Autodesk Inventor part; units mm, degrees
ref_plane "YZ Plane" through (0, 0, 0) normal (1, 0, 0) x (0, 1, 0)
ref_plane "XZ Plane" through (0, 0, 0) normal (0, 1, 0) x (-1, 0, 0)
ref_plane "XY Plane" through (0, 0, 0) normal (0, 0, 1) x (1, 0, 0)
sketch "Schizzo1" plane through (0, 0, 0) normal (0, 0, 1) x (1, 0, 0)
  line L0 (9, 6) -> (9, -6)
  line L1 (6, -9) -> (-6, -9)
  line L2 (-9, -6) -> (-9, 6)
  line L3 (-6, 9) -> (6, 9)
  arc A0 (-6, 9) -> (-9, 6) centre (-6, 6) ccw
  arc A1 (-9, -6) -> (-6, -9) centre (-6, -6) ccw
  arc A2 (6, -9) -> (9, -6) centre (6, -6) ccw
  arc A3 (9, 6) -> (6, 9) centre (6, 6) ccw
  point P0 (0, 0)
  point P1 (0, 0)
  point P2 (9, 9)
  point P3 (9, -9)
  point P4 (-9, -9)
  point P5 (-9, 9)
  dimension "d0" = 18
  dimension "d72" = 3
extrude "Estrusione1" add sketch "Schizzo1" against normal blind 40
sketch "Schizzo2" plane through (0, 0, 0) normal (0, 0, 1) x (1, 0, 0)
  line L0 (18.5, -15) -> (-18.5, -15)
  line L1 (-18.5, -15) -> (-18.5, 15)
  line L2 (-18.5, 15) -> (18.5, 15)
  line L3 (18.5, 15) -> (18.5, -15)
  line L4 (18.5, -15) -> (-18.5, 15) construction
  line L5 (-18.5, -15) -> (18.5, 15) construction
  point P0 (0, 0)
  dimension "d3" = 30
  dimension "d4" = 37
extrude "Estrusione2" add sketch "Schizzo2" along normal blind 50
sketch "Schizzo3" plane through (-18.5, 15, 0) normal (0, 1, 0) x (1, 0, 0)
  line L0 (18.5, 0) -> (18.5, -22.5)
  line L1 (18.5, 0) -> (41, 0) construction
  circle A0 centre (18.5, -22.5) radius 12.5
  dimension "d7" = 22.5
  dimension "d8" = 90
  dimension "d9" = 25
extrude "Estrusione3" cut sketch "Schizzo3" against normal blind 30
sketch "Schizzo4" plane through (-18.5, 15, 0) normal (0, 1, 0) x (1, 0, 0)
  circle A0 centre (18.5, -22.5) radius 12.5
  line L0 (18.5, -22.5) -> (18.5, -34.5)
  line L1 (18.5, -34.5) -> (15, -34.5)
  line L2 (18.5, -34.5) -> (22, -34.5)
  line L3 (0, -50) -> (37, -50)
  line L4 (18.5, -50) -> (20.5, -50)
  line L5 (18.5, -50) -> (20.5, -50) construction
  line L6 (20.5, -50) -> (20.5, -34.5)
  line L7 (18.5, -50) -> (16.5, -50)
  line L8 (16.5, -50) -> (20.5, -50)
  line L9 (20.5, -50) -> (20.5, -34.5)
  line L10 (20.5, -34.5) -> (16.5, -34.5)
  line L11 (16.5, -34.5) -> (16.5, -50)
  point P0 (18.5, 0)
  point P1 (16.5, -34.839)
  point P2 (20.5, -34.839)
  dimension "d12" = 12
  dimension "d13" = 2
  dimension "d14" = 0
  dimension "d15" = 2
extrude "Estrusione4" cut sketch "Schizzo4" against normal blind 30 contours A0 L6 L3 L11
sketch "Schizzo5" plane through (-18.5, 15, 0) normal (0, 1, 0) x (1, 0, 0)
  arc A0 (20.5, -34.839) -> (16.5, -34.839) centre (18.5, -22.5) ccw
  circle A1 centre (18.5, -22.5) radius 18.5
  line L0 (20.5, -50) -> (20.5, -34.839)
  line L1 (20.5, -50) -> (26.5, -50)
  line L2 (37, -50) -> (20.5, -50)
  line L3 (26.5, -50) -> (26.5, -39.1808)
  line L4 (37, 0) -> (37, -50)
  line L5 (26.5, -50) -> (37, -50)
  line L6 (37, -50) -> (37, -22.5)
  point P0 (18.5, 0)
  dimension "d18" = 37
  dimension "d19" = 6
extrude "Estrusione5" cut sketch "Schizzo5" against normal blind 30 contours A1 L4 L2 L3
sketch "Schizzo6" plane through (-18.5, 15, 0) normal (0, 1, 0) x (1, 0, 0)
  line L0 (16.5, -50) -> (0, -50)
  line L1 (16.5, -50) -> (10.5, -50)
  arc A0 (20.5, -34.839) -> (16.5, -34.839) centre (18.5, -22.5) ccw
  circle A1 centre (18.5, -22.5) radius 18.5
  line L2 (0, 0) -> (0, -50)
  line L3 (10.5, -50) -> (0, -50)
  line L4 (0, -50) -> (0, -22.5)
  line L5 (10.5, -50) -> (10.5, -39.1808)
  line L6 (10.5, -50) -> (21.3192, -50) construction
  point P0 (18.5, 0)
  dimension "d22" = 6
  dimension "d23" = 37
  dimension "d24" = 90
extrude "Estrusione6" cut sketch "Schizzo6" against normal blind 30 contours L0 L2 A1 L5
sketch "Schizzo7" plane through (-18.5, 15, 0) normal (0, 1, 0) x (1, 0, 0)
  arc A0 (20.5, -34.839) -> (16.5, -34.839) centre (18.5, -22.5) ccw
  line L0 (0, 0) -> (0, -22.5)
  circle A1 centre (18.5, -22.5) radius 18.5
  line L1 (18.5, 0) -> (4.5, 0)
  line L2 (37, 0) -> (0, 0)
  line L3 (18.5, 0) -> (32.5, 0) construction
  line L4 (4.5, 0) -> (4.5, -10.4066)
  dimension "d73" = 37
  dimension "d74" = 14
  dimension "d75" = 180
  dimension "d76" = 90
extrude "Estrusione7" cut sketch "Schizzo7" against normal blind 30 contours L2 L4 A1 L0
sketch "Schizzo8" plane through (0, 15, 22.5) normal (0, 1, 0) x (1, 0, 0)
  line L0 (-6, 22.5) -> (6, 22.5)
  arc A0 (2, -12.339) -> (-2, -12.339) centre (0, 0) ccw
  circle A1 centre (0, 0) radius 18.5
  line L1 (0, 22.5) -> (14, 22.5)
  line L2 (0, 22.5) -> (14, 22.5) construction
  line L3 (14, 22.5) -> (14, 12.0934)
  line L4 (-18.5, 22.5) -> (18.5, 22.5)
  line L5 (14, 22.5) -> (18.5, 22.5)
  line L6 (18.5, 22.5) -> (18.5, 0)
  point P0 (-9, 22.5)
  point P1 (9, 22.5)
  point P2 (-14, 22.5)
  dimension "d35" = 37
  dimension "d36" = 14
  dimension "d38" = 90
extrude "Estrusione8" cut sketch "Schizzo8" against normal blind 30 contours A1 L3 L4 L6
sketch "Schizzo10" plane through (0, 0, 50) normal (0, 0, 1) x (1, 0, 0)
  line L0 (-8, 15) -> (-8, -15)
  line L1 (-8, -15) -> (8.0102, -15)
  line L2 (8.0102, -15) -> (8.0102, 15)
  line L3 (8.0102, 15) -> (-8, 15)
  line L4 (-8, 15) -> (-8, -15)
  line L5 (-8, -15) -> (-2, -15)
  line L6 (2, 15) -> (2, -15)
  line L7 (-2, -15) -> (2, -15)
  line L8 (2, -15) -> (2, 15)
  line L9 (2, 15) -> (-2, 15)
  line L10 (-2, 15) -> (-2, -15)
  point P0 (0, 0)
  point P1 (-8, 15)
extrude "Estrusione9" add sketch "Schizzo10" along normal blind 5 contours L3 L10 L1 L0 | L3 L2 L1 L6
sketch "Schizzo11" plane through (-8, -15, 39.1808) normal (-1, 0, 0) x (0, 0, 1)
  line L0 (15.8192, 0) -> (15.8192, 30)
  line L1 (15.8192, 15) -> (7.8192, 15)
  line L2 (7.8192, 15) -> (7.8192, 22)
  line L3 (7.8192, 15) -> (7.8192, 8)
  line L4 (10.8192, 0) -> (10.8192, 30)
  line L5 (7.8192, 15) -> (14.8192, 15) construction
  point P0 (-39.1808, 15)
  dimension "d43" = 8
  dimension "d44" = 7
  dimension "d45" = 7
  dimension "d46" = 90
hole "Foro1" at (-8, 7, 47) at (-8, -7, 47) direction (1, 0, 0) diameter 5 end through all
sketch "Schizzo14" plane through (0, 0, 0) normal (0, 0, -1) x (-1, 0, 0)
  line L0 (10.5, 8.5) -> (10.5, -8.5)
  line L1 (8.5, -10.5) -> (-8.5, -10.5)
  line L2 (-10.5, -8.5) -> (-10.5, 8.5)
  line L3 (-8.5, 10.5) -> (8.5, 10.5)
  line L4 (13, 11) -> (13, -11)
  line L5 (11, -13) -> (-11, -13)
  line L6 (-13, -11) -> (-13, 11)
  line L7 (-11, 13) -> (11, 13)
  arc A0 (-8.5, 10.5) -> (-10.5, 8.5) centre (-8.5, 8.5) ccw
  arc A1 (8.5, -10.5) -> (10.5, -8.5) centre (8.5, -8.5) ccw
  arc A2 (-10.5, -8.5) -> (-8.5, -10.5) centre (-8.5, -8.5) ccw
  arc A3 (10.5, 8.5) -> (8.5, 10.5) centre (8.5, 8.5) ccw
  arc A4 (-11, 13) -> (-13, 11) centre (-11, 11) ccw
  arc A5 (13, 11) -> (11, 13) centre (11, 11) ccw
  arc A6 (11, -13) -> (13, -11) centre (11, -11) ccw
  arc A7 (-13, -11) -> (-11, -13) centre (-11, -11) ccw
  point P0 (0, 0)
  point P1 (0, 0)
  point P2 (10.5, 10.5)
  point P3 (10.5, -10.5)
  point P4 (-10.5, -10.5)
  point P5 (-10.5, 10.5)
  point P6 (0, 0)
  point P7 (13, 13)
  point P8 (13, -13)
  point P9 (-13, -13)
  point P10 (-13, 13)
  dimension "d77" = 21
  dimension "d78" = 26
  dimension "d79" = 2
extrude "Estrusione10" add sketch "Schizzo14" along normal blind 40
sketch "Schizzo15" plane through (0, 15, 22.5) normal (0, 1, 0) x (1, 0, 0)
  line L0 (-13, 12.5) -> (13, 12.5)
  line L1 (13, 12.5) -> (13, 17.5)
  line L2 (13, 17.5) -> (-13, 17.5)
  line L3 (-13, 17.5) -> (-13, 12.5)
  arc A0 (2, -12.339) -> (-2, -12.339) centre (0, 0) ccw
  point P0 (0, 22.5)
  point P1 (0, 12.5)
  dimension "d82" = 26
  dimension "d83" = 5
extrude "Estrusione11" [suppressed]
sketch "Schizzo16" plane through (-11, -13, 0) normal (0, -1, 0) x (1, 0, 0)
  line L0 (11, 0) -> (11, -13)
  dimension "d88" = 13
hole "Foro4" at (0, -13, -13) direction (0, 1, 0) diameter 5.5 depth 26
sketch "Schizzo17" plane through (13, -11, 0) normal (1, 0, 0) x (0, 0, -1)
  line L0 (0, 11) -> (27, 11)
  dimension "d96" = 27
hole "Foro5" at (13, 0, -27) direction (-1, 0, 0) diameter 5.5 depth 26
properties part number "5_Connettore_sup_inf"
Work out the finished part from the listing and answer in its coordinate system (mm). A direction names the side the tool comes from. Give positions to 0.01 mm unless a question says otherwise; leave off trailing zeros. Order: outer loops, then holes, each group sorted by start corner. A loop starts at its lowest first (then second) coordinate and runs counter-clockwise, first axis right, second up. Notation, with made-up numbers: M 41,39.25 L 95,39.25 A34 ccw 95,78.25 Z; hole C -12.5,-28.5 d7. An arc over 180 degrees is marked long. Return JSON: item names as keys, results as strings.
1) Section A-A, the plane x = 0 is taken. Give the number of separate pieces and of enclosed holes in the cut face, plus the area to 3 significant figures.
Resolved:
{"separate pieces": "4", "enclosed holes": "1", "area": "1,070 mm^2"}
2) Each of these flat-tipped pins is pushed along its axis until it touches: pin 1 (7 mm diameter, centred on y = 0, z = -27, fed in from +X); pin 2 (5 mm diameter, centred on y = -2, z = -20, fed in from -X); pin 3 (2.5 mm diameter, centred on y = -2.5, z = 53.5, fed in from +X); pin 4 (8 mm diameter, centred on x = -7.5, y = 9.5, fed in from -Z). Where does it stop, or does it pass through?
Resolved:
{"pin 1": "x = 13", "pin 2": "x = -13", "pin 3": "x = 8.01", "pin 4": "z = -40"}
3) Section C-C, the plane x = -4.5 is taken. Write down the section's boundary in (y, z).
Resolved:
{"outline": "M -15,0 L -13,0 L -13,-40 L -10.5,-40 L -10.5,0 L -9,0 L -9,-40 L 9,-40 L 9,0 L 10.5,0 L 10.5,-40 L 13,-40 L 13,0 L 15,0 L 15,10.84 L -15,10.84 Z; M -15,34.16 L 15,34.16 L 15,55 L -15,55 Z; hole C -7,47 d5; hole C 0,-27 d5.5; hole C 7,47 d5"}
4) Straight lines are drawn through the part: line 1 along Y through (x, z) = (0, -21.5); line 2 along Y through (x, z) = (-4.7, 47); line 3 along X through (y, z) = (6, -13). For each, find the intervals that lie inside material, in ascending order. Write a range as [from, to].
Resolved:
{"line 1": "[-13, -10.5], [-9, 9], [10.5, 13]", "line 2": "[-15, -9.5], [-4.5, 4.5], [9.5, 15]", "line 3": "[-13, -10.5], [-9, -2.75], [2.75, 9], [10.5, 13]"}
5) Section B-B, the plane z = 22.5 is taken. Write down the section's boundary in (x, y).
Resolved:
{"outline": "M -18.5,-15 L -12.5,-15 L -12.5,15 L -18.5,15 Z; M 12.5,-15 L 18.5,-15 L 18.5,15 L 12.5,15 Z"}
6) A tool of negligible diameter and unlimited length cuts with its end or side. For faces 1 (the flat face through (2, 0, 45)), 2 (the flat face through (-10.5, 0, -20)), 3 (the cylindrical face through (-0.126, -0.121, -24.253)), from which of +Z, -Z, +X, -X, +Y, -Y can it reach the whole face along a straight path? Write none if from no direction.
Resolved:
{"face 1": "+Z, +Y, -Y", "face 2": "-Z", "face 3": "+X, -X"}
7) For a pull along X with two mould halves and no side action, classify faces 4 (the cylindrical face through (0.52, 0.21, 10.01)), 5 (the flat face through (0, -9, -20)), 6 (the cylindrical face through (-12.43, -12.4, -19.72)), 7 (the cylindrical face through (5.04, 7.96, 49.31)) as +X half, -X half, draft (parallel to the pull), parting line (faces both ways), or undercut.
Resolved:
{"face 4": "undercut", "face 5": "undercut", "face 6": "-X half", "face 7": "draft"}
